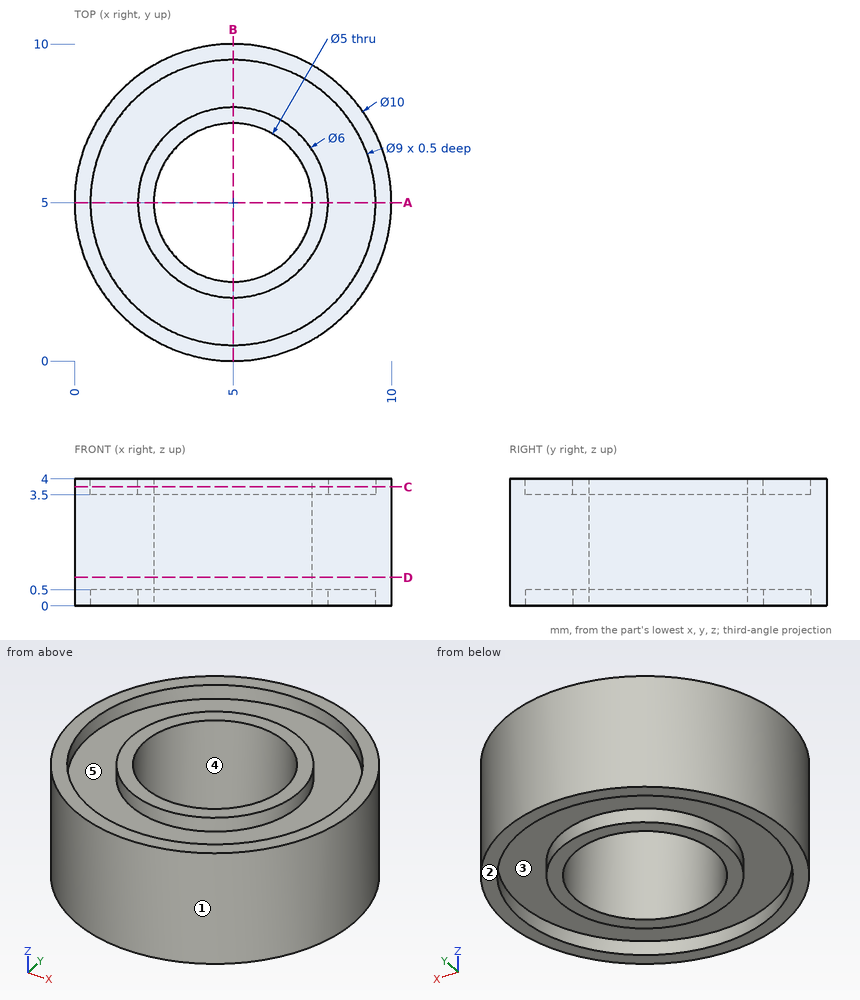
Source: three-view drawing plus pictorial views. Frame: mm from the lowest corner of the part. A direction names the side the tool comes from. Round coordinates to 2 decimals unless told otherwise and drop trailing zeros. Loops run counter-clockwise (first coordinate to the right, second up) from the corner with the lowest first, then second, coordinate; pieces in that order, holes last. Notation, with made-up numbers: M 87.5,18 L 123.5,18 A6 ccw 123.5,25 Z; hole C 13.5,27.5 d6. An arc over 180 degrees is marked long. Put each result on its own line as item: value.
(1) Ray query, line 1 (Y direction, x = 5, z = 3.7); line 2 (X direction, y = 3, z = 3.8); line 3 (X direction, y = 5.25, z = 0.35). Return the intervals inside material, ascending. Write a range as [from, to].
Solutions:
line 1: [0, 0.5], [2, 2.5], [7.5, 8], [9.5, 10]
line 2: [0.42, 0.97], [2.76, 3.5], [6.5, 7.24], [9.03, 9.58]
line 3: [0.01, 0.51], [2.01, 2.51], [7.49, 7.99], [9.49, 9.99]
(2) Section D-D, the plane z = 0.9. Return loops of the section in (x, y).
Solutions:
outline: C 5,5 d10; hole C 5,5 d5
(3) Section A-A, the plane y = 5. Return loops of the section in (x, z).
Solutions:
outline: M 0,0 L 0.5,0 L 0.5,0.5 L 2,0.5 L 2,0 L 2.5,0 L 2.5,4 L 2,4 L 2,3.5 L 0.5,3.5 L 0.5,4 L 0,4 Z; M 7.5,0 L 8,0 L 8,0.5 L 9.5,0.5 L 9.5,0 L 10,0 L 10,4 L 9.5,4 L 9.5,3.5 L 8,3.5 L 8,4 L 7.5,4 Z
(4) Section C-C, the plane z = 3.75. Return loops of the section in (x, y).
Solutions:
outline: C 5,5 d10; C 5,5 d6; hole C 5,5 d9; hole C 5,5 d5
(5) First-contact query: pin 1 (1 mm diameter, centred on x = 8, z = 2.5, fed in from -Y); pin 2 (2 mm diameter, centred on x = 7, z = 2.5, fed in from +Y). Flat tips, straight axial feed; report the tip coordinate or a pass-through.
Solutions:
pin 1: y = 0.67
pin 2: y = 9.9
(6) Pull-direction query (X, two-part tool) for the marked faces 1, 2 and 3; classes: released by +X, released by -X, zero draft, split by the parting line, or undercut.
Solutions:
face 1: split by the parting line
face 2: zero draft
face 3: undercut
(7) Access query for the marked faces 4 and 5. Directions: +Z, -Z, +X, -X, +Y, -Y. A direction counts if a zero-diameter tool reaches every point of the face in a straight line with its end or side. Return the directions, or none.
Solutions:
face 4: +Z, -Z
face 5: +Z
